Can you work these out from the drawing? Everything is in mm from the part's minimum corner. A direction names the side the tool comes from. Give positions to 0.01 mm unless a question says otherwise; leave off trailing zeros. Loops run counter-clockwise (first coordinate to the right, second up) from the corner with the lowest first, then second, coordinate; pieces in that order, holes last. Notation, with made-up numbers: (87, 32) -> (146, 32) arc R21 cw to (146, 42) -> close; hole circle Ø3 at (69.5, -39). An arc over 180 degrees is marked (long way). Write item = value, one per line. Start each with the question number.
1) I want a section at C-C (x = 87). List the corners of the cut face in (y, z) for me.
2) I want a section at B-B (y = 44.45). List the corners of the cut face in (x, z) for me, and give its area (3 significant figures).
3) I want a section at A-A (z = 24). List the corners of the cut face in (x, y) for me.
4) I want a section at D-D (y = 82). List the corners of the cut face in (x, z) for me, and give its area (3 significant figures).
5) I'm going to push flat-ended pins straight in: pin 1 Ø4 at (x, z) = (101, 36.5) entering from +Y; pin 2 Ø4 at (x, z) = (83, 39) entering from -Y; pin 3 Ø21 at (x, y) = (75.5, 6) entering from +Z. Where does each tip first touch, or does it pass through?
6) On a 3-axis mill with a long thin cutter (end or side, diameter ignored), from which of +Z, -Z, +X, -X, +Y, -Y can I reach the whole of each face in a straight line? I mean the marked faces 1, 2, 3 and 4. Say none if no direction works.
7) If we mould it in two halves opening along Y, with no side actions, what happens to the marked faces 5, 6, 7 and 8? For each: +Y half, -Y half, draft (parallel to the pull), parting line (faces both ways), or undercut.
8) I need wall thicknesses on probe 1 along X at (y, z) = (44.45, 36.25); probe 2 along X at (y, z) = (44, 36); probe 3 along Y at (x, z) = (69, 2.5). Which ranges of each line are inside material? Lowest first, please. Write a range as from..to.
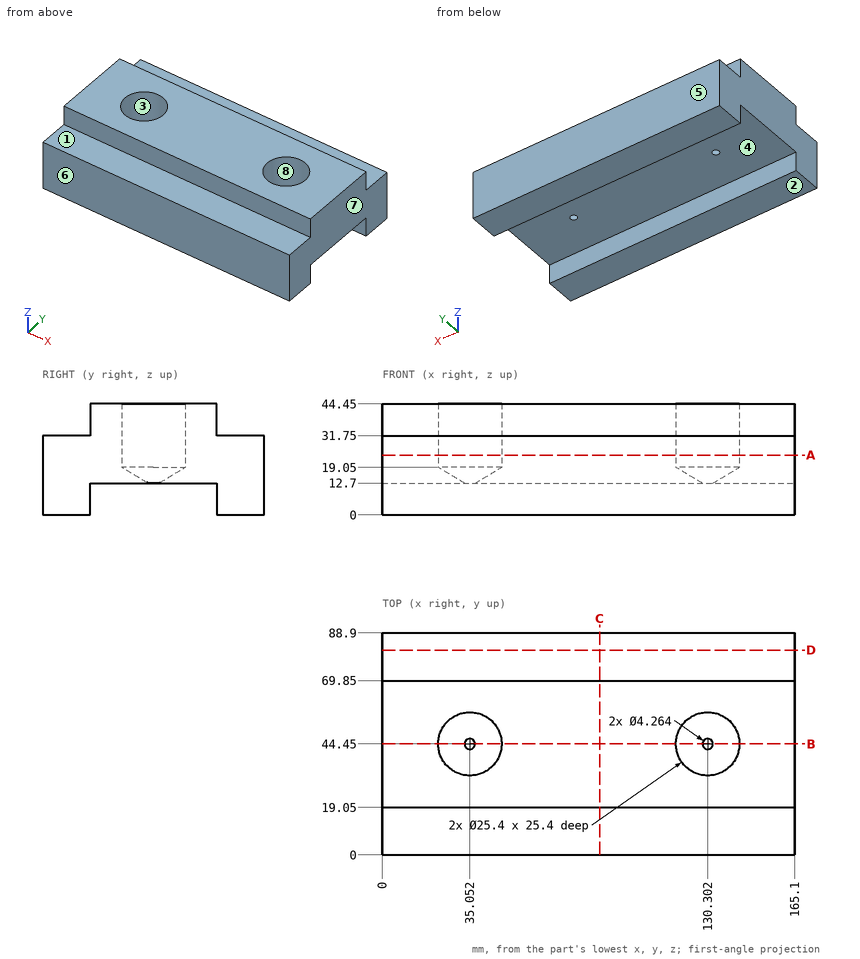
Answer list:
q1.outline = (0, 0) -> (19.05, 0) -> (19.05, 12.7) -> (69.85, 12.7) -> (69.85, 0) -> (88.9, 0) -> (88.9, 31.75) -> (69.85, 31.75) -> (69.85, 44.45) -> (19.05, 44.45) -> (19.05, 31.75) -> (0, 31.75) -> close
q2.outline = (0, 12.7) -> (32.92, 12.7) -> (22.35, 19.05) -> (22.35, 44.45) -> (0, 44.45) -> close; (37.18, 12.7) -> (128.17, 12.7) -> (117.6, 19.05) -> (117.6, 44.45) -> (47.75, 44.45) -> (47.75, 19.05) -> close; (132.43, 12.7) -> (165.1, 12.7) -> (165.1, 44.45) -> (143, 44.45) -> (143, 19.05) -> close
q2.area = 3,760 mm^2
q3.outline = (0, 0) -> (165.1, 0) -> (165.1, 88.9) -> (0, 88.9) -> close; hole circle Ø25.4 at (35.05, 44.45); hole circle Ø25.4 at (130.3, 44.45)
q4.outline = (0, 0) -> (165.1, 0) -> (165.1, 31.75) -> (0, 31.75) -> close
q4.area = 5,240 mm^2
q5.pin_1 = 69.85
q5.pin_2 = 19.05
q5.pin_3 = 31.75
q6.face_1 = +Z, +X, -X, -Y
q6.face_2 = -Z, +X, -X, +Y, -Y
q6.face_3 = +Z
q6.face_4 = -Z, +X, -X
q7.face_5 = +Y half
q7.face_6 = -Y half
q7.face_7 = draft
q7.face_8 = undercut
q8.probe_1 = 0..22.35, 47.75..117.6, 143..165.1
q8.probe_2 = 0..22.36, 47.74..117.61, 142.99..165.1
q8.probe_3 = 0..19.05, 69.85..88.9
